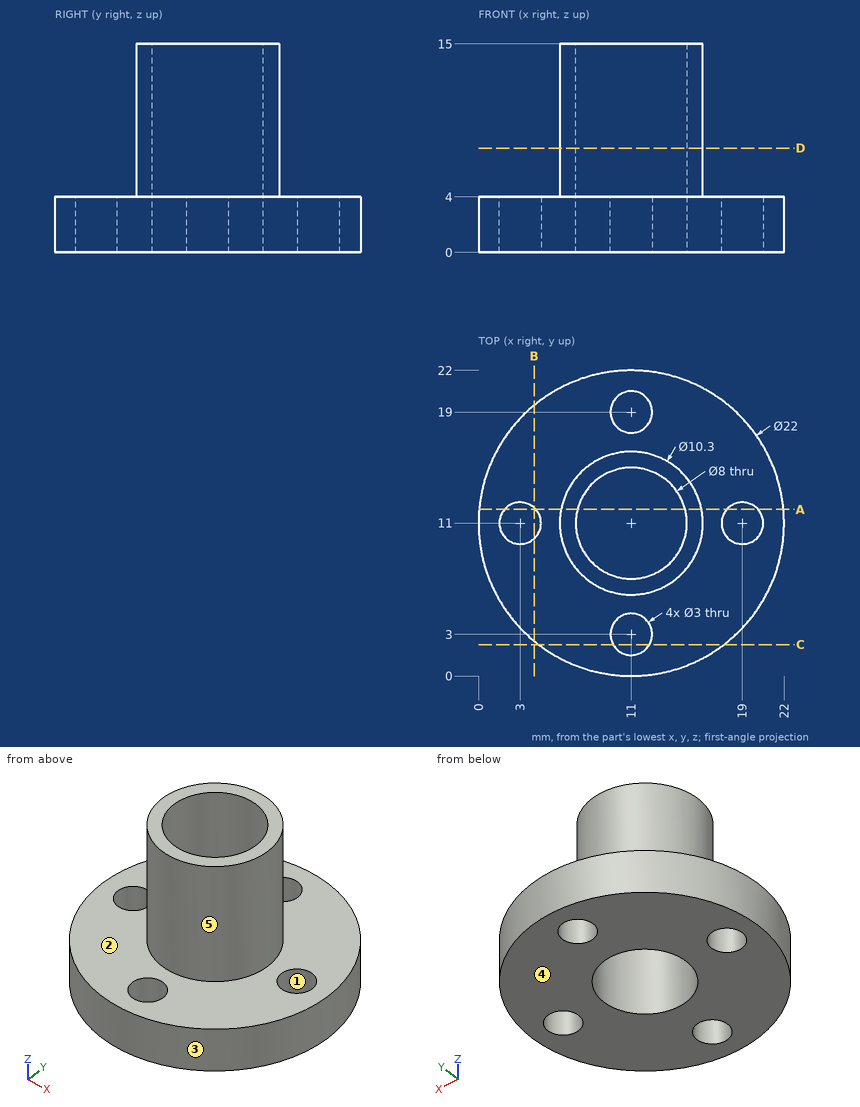
Can you work these out from the drawing? Everything is in mm from the part's minimum corner. A direction names the side the tool comes from. Round coordinates to 2 decimals unless told otherwise and drop trailing zeros. Order: outer loops, then holes, each group sorted by start corner. A loop starts at its lowest first (then second) coordinate and runs counter-clockwise, first axis right, second up. Notation, with made-up numbers: (-30, 60) -> (-19, 60) arc R20 ccw to (-19, 85) -> close; hole circle Ø11 at (-1, 31.25). An arc over 180 degrees is marked (long way). Return JSON: item names as keys, results as strings. Group by question number.
1. Which directions (+Z, -Z, +X, -X, +Y, -Y) give clear straight access to the entire face, cutting with the end or side of a thin tool? Please do the marked faces 4 and 5.
2. If we section it at D-D, the plane z = 7.5: Write out the boundary of the cut face in (x, y), then the cut area to 3 significant figures.
3. If we section it at C-C, the plane y = 2.25: Write out the boundary of the cut face in (x, z).
4. If we section it at A-A, the plane y = 12: Write out the boundary of the cut face in (x, z), then the cut area to 3 significant figures.
5. I need wall thicknesses on line 1 (Y direction, x = 11, z = 0.85); line 2 (Y direction, x = 11, z = 8.75); line 3 (Z direction, x = 2, y = 13.25). Which ranges of each line are inside material? Lowest first, please. Write a range as [from, to].
6. We'd pull the mould along Y, two halves only. Please class the marked faces 1, 2 and 3: released by +Y, released by -Y, zero draft, split by the parting line, or undercut.
7. If we section it at B-B, the plane x = 4: Write out the boundary of the cut face in (y, z).
8. Will these pins go through, and if not, where does the flat tip stop? pin 1 (4 mm diameter, centred on x = 11, y = 19, fed in from +Z); pin 2 (8 mm diameter, centred on x = 19.5, z = 3.5, fed in from +Y); pin 3 (1 mm diameter, centred on y = 15.5, z = 5, fed in from +X).
Output values:
{
 "1": {"face 4": "-Z, +X, -X, +Y, -Y", "face 5": "+Z"},
 "2": {"outline": "circle Ø10.3 at (11, 11); hole circle Ø8 at (11, 11)", "area": "33.1 mm²"},
 "3": {"outline": "(4.33, 0) -> (9.7, 0) -> (9.7, 4) -> (4.33, 4) -> close; (12.3, 0) -> (17.67, 0) -> (17.67, 4) -> (12.3, 4) -> close"},
 "4": {"outline": "(0.05, 0) -> (1.88, 0) -> (1.88, 4) -> (0.05, 4) -> close; (4.12, 0) -> (7.13, 0) -> (7.13, 15) -> (5.95, 15) -> (5.95, 4) -> (4.12, 4) -> close; (14.87, 0) -> (17.88, 0) -> (17.88, 4) -> (16.05, 4) -> (16.05, 15) -> (14.87, 15) -> close; (20.12, 0) -> (21.95, 0) -> (21.95, 4) -> (20.12, 4) -> close", "area": "64.7 mm²"},
 "5": {"line 1": "[0, 1.5], [4.5, 7], [15, 17.5], [20.5, 22]", "line 2": "[5.85, 7], [15, 16.15]", "line 3": "[0, 4]"},
 "6": {"face 1": "undercut", "face 2": "zero draft", "face 3": "split by the parting line"},
 "7": {"outline": "(2.51, 0) -> (9.88, 0) -> (9.88, 4) -> (2.51, 4) -> close; (12.12, 0) -> (19.49, 0) -> (19.49, 4) -> (12.12, 4) -> close"},
 "8": {"pin 1": "z = 4", "pin 2": "y = 21.04", "pin 3": "x = 14.24"}
}
